Check sheet for the drawn part. Datum: minimum x, y, z corner. Units: mm. A direction names the side the tool comes from. Give positions to 0.01 mm unless a question says otherwise; leave off trailing zeros. Write each loop counter-clockwise with the first axis right and the second up, starting at its lowest first coordinate (ties: lowest second). Pieces come first, ordered by that corner, then holes. Notation, with made-up numbers: (25, 40) -> (62, 40) arc R35 ccw to (62, 72) -> close; hole circle Ø5 at (19.5, 85.25). An arc over 180 degrees is marked (long way). Answer as CSV lines item,"result". Start each with the question number.
1) Material ranges on L1, parallel to X at y = 15.75, z = 25; L2, parallel to Z at x = 17, y = 8.25; L3, parallel to X at y = 19.25, z = 85, recorded low to high.
2) Tool access check on the marked faces 4 and 5. Record the directions out of +Z, -Z, +X, -X, +Y, -Y that give a thin tool (end or side, any length) a straight path to the whole face; none if there is none.
3) Sectioned sample at A-A on y = 16.25. Give the number of separate pieces and of enclosed holes in the cut face, and give its area (3 significant figures).
4) Mould release check, pull along Z, two halves, no side actions. Record for the marked faces 1, 2 and 3: released by +Z, released by -Z, zero draft, split by the parting line, or undercut.
5) Sectioned sample at C-C on z = 51. Record the cut outline in (x, y), and give its area (3 significant figures).
6) Sectioned sample at B-B on x = 17. Record the cut outline in (y, z), and give its area (3 significant figures).
7) Sectioned sample at D-D on x = 75.5. Record the cut outline in (y, z).
8) Gauge pin test, flat ends, axial feed: pin 1 Ø6.5 at (x, z) = (47, 29.5) entering from +Y; pin 2 Ø1.5 at (y, z) = (13.5, 49.5) entering from -X. Record the tip position at first contact, or that the pin passes through.
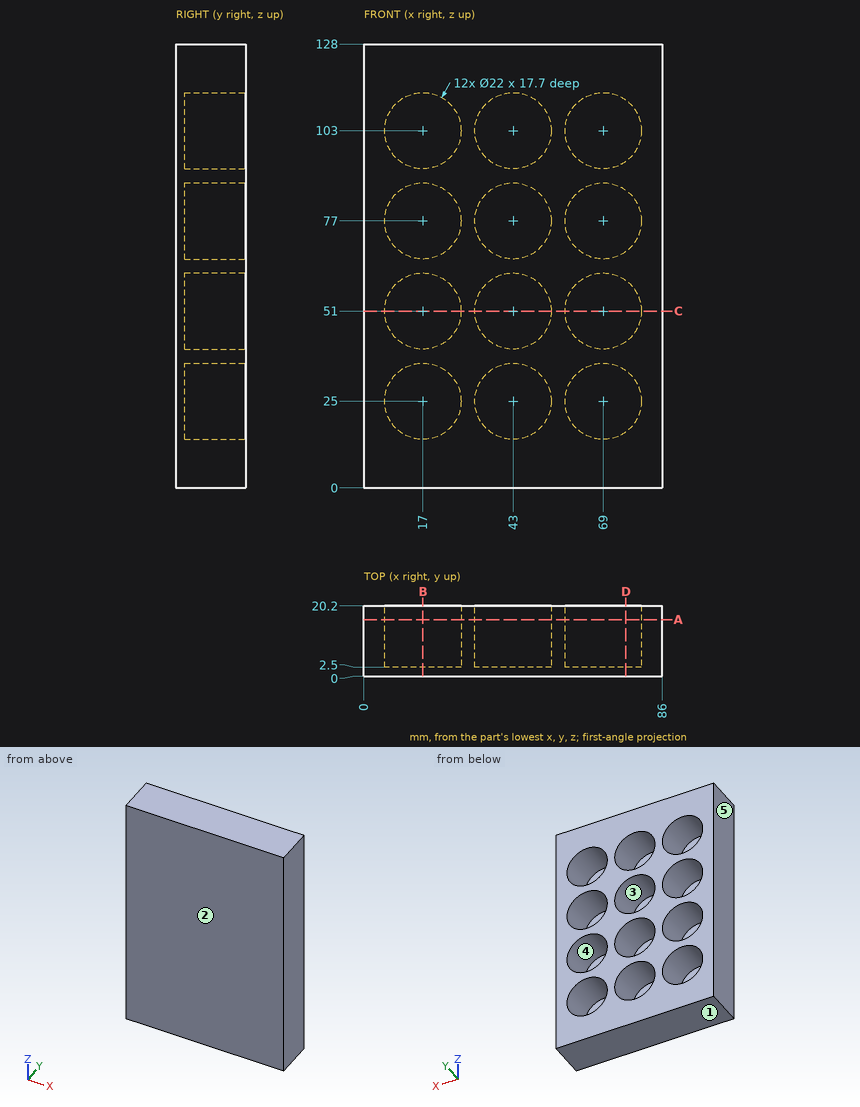
Ans:
1,L1,"x = 0 to 6, 28 to 32, 54 to 58, 80 to 86"
1,L2,"z = 0 to 14, 36 to 40, 62 to 66, 88 to 92, 114 to 128"
1,L3,"x = 0 to 9.45, 24.55 to 35.45, 50.55 to 61.45, 76.55 to 86"
2,face 4,"+Y"
2,face 5,"+Z, -Z, -X, +Y, -Y"
3,separate pieces,"1"
3,enclosed holes,"12"
3,area,"6,450 mm²"
4,face 1,"released by -Z"
4,face 2,"zero draft"
4,face 3,"undercut"
5,outline,"(0, 0) -> (86, 0) -> (86, 20.2) -> (80, 20.2) -> (80, 2.5) -> (58, 2.5) -> (58, 20.2) -> (54, 20.2) -> (54, 2.5) -> (32, 2.5) -> (32, 20.2) -> (28, 20.2) -> (28, 2.5) -> (6, 2.5) -> (6, 20.2) -> (0, 20.2) -> close"
5,area,"569 mm²"
6,outline,"(0, 0) -> (20.2, 0) -> (20.2, 14) -> (2.5, 14) -> (2.5, 36) -> (20.2, 36) -> (20.2, 40) -> (2.5, 40) -> (2.5, 62) -> (20.2, 62) -> (20.2, 66) -> (2.5, 66) -> (2.5, 88) -> (20.2, 88) -> (20.2, 92) -> (2.5, 92) -> (2.5, 114) -> (20.2, 114) -> (20.2, 128) -> (0, 128) -> close"
6,area,"1,030 mm²"
7,outline,"(0, 0) -> (20.2, 0) -> (20.2, 16.13) -> (2.5, 16.13) -> (2.5, 33.87) -> (20.2, 33.87) -> (20.2, 42.13) -> (2.5, 42.13) -> (2.5, 59.87) -> (20.2, 59.87) -> (20.2, 68.13) -> (2.5, 68.13) -> (2.5, 85.87) -> (20.2, 85.87) -> (20.2, 94.13) -> (2.5, 94.13) -> (2.5, 111.87) -> (20.2, 111.87) -> (20.2, 128) -> (0, 128) -> close"
8,pin 1,"stops at y = 2.5"
8,pin 2,"stops at x = 0"
